Drawing for the job (mm, zero at the part's lowest x, y, z). A direction names the side the tool comes from. Give positions to 0.01 mm unless a question says otherwise; leave off trailing zeros. Loops run counter-clockwise (first coordinate to the right, second up) from the corner with the lowest first, then second, coordinate; pieces in that order, holes last.
1) Band-saw the part on C-C on y = 17. List the corners of the cut face in (x, z), then the cut area to 3 significant figures.
2) Band-saw the part on B-B on z = 21. List the corners of the cut face in (x, y).
3) Flat gauge pins, fed straight in: P1, Ø12.5, axis at x = 19.5, z = 12.5, coming from the -Y side; P2, Ø9.5, axis at y = 35, z = 13.5, coming from the +X side; P3, Ø0.8, axis at x = 44.5, z = 25.5, coming from the -Y side; P4, Ø2, axis at x = 41, y = 6, coming from the +Z side. Where does each tip first touch, or does it go through?
4) 3-axis set-ups, long thin cutter, end or side, ignore diameter. For the marked faces 1 and 2: which of +Z, -Z, +X, -X, +Y, -Y reach the whole face in a straight line?
5) Band-saw the part on A-A on x = 11.5. List the corners of the cut face in (y, z).
6) Wall check: line 1 (Z direction, x = 24.5, y = 14); line 2 (Y direction, x = 17.5, z = 22.5). Give the ranges that are in metal, low to high.
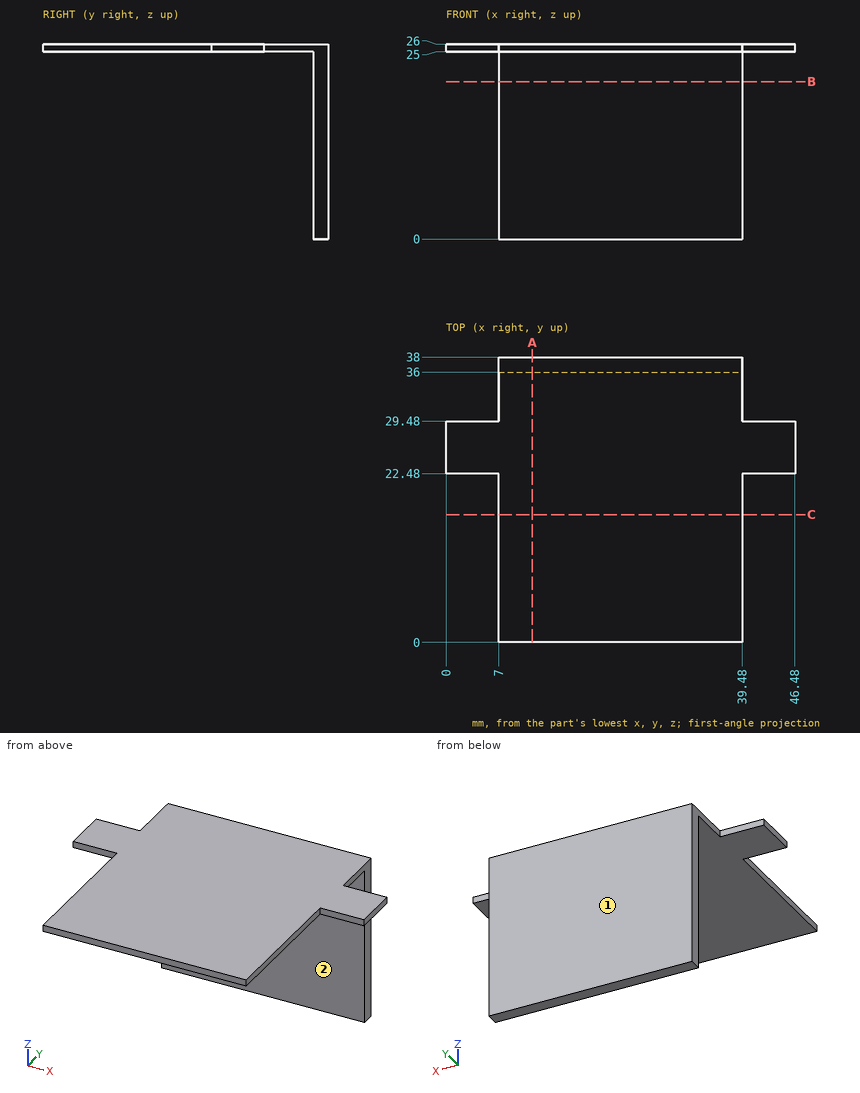
Findings below:
1. outline: (7, 25) - (39.48, 25) - (39.48, 26) - (7, 26) - close
1. area: 32.5 mm2
2. outline: (7, 36) - (39.48, 36) - (39.48, 38) - (7, 38) - close
3. P1: stops at y = 36
3. P2: stops at x = 39.48
3. P3: stops at y = 22.48
3. P4: passes through
4. face 1: +Z, -Z, +X, -X, +Y
4. face 2: -Z, +X, -X, -Y
5. outline: (0, 25) - (36, 25) - (36, 0) - (38, 0) - (38, 26) - (0, 26) - close
6. line 1: z = 25 to 26
6. line 2: y = 36 to 38
